For this review, use the dimensioned drawing (mm, ordinates from the lowest corner) and the shaded views. A direction names the side the tool comes from. Round coordinates to 2 decimals unless told otherwise and drop trailing zeros. Order: outer loops, then holes, each group sorted by start corner. A loop starts at its lowest first (then second) coordinate and runs counter-clockwise, first axis right, second up. Notation, with made-up numbers: (2, 18) - (39, 18) arc R29 ccw to (39, 48) - close; hole circle Ø11 at (30.25, -16.75). An arc over 180 degrees is marked (long way). Use CSV: the item, a comma, the result in double quotes. Start each with the question number.
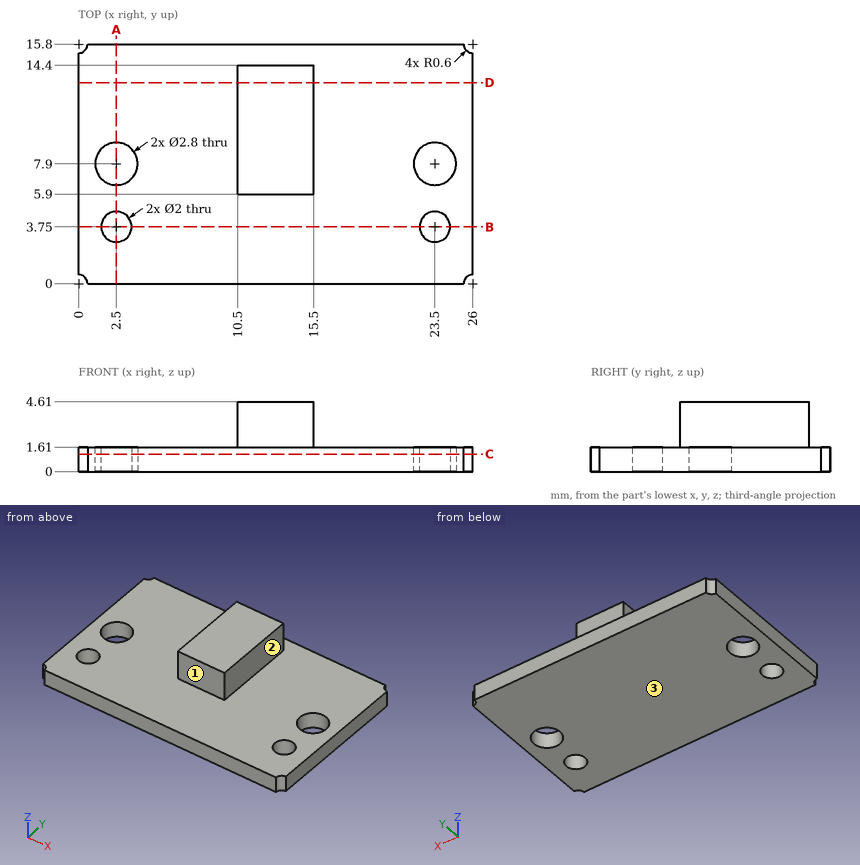
Q1. Take a section at C-C (z = 1.15). State the section outline as (x, y) points, plus the area to 3 significant figures.
Q2. For L1, parallel to Y at x = 23.5, z = 1.35; L2, parallel to Z at x = 5.25, y = 8.5; L3, parallel to X at y = 14, z = 4.3, list the stretches that pass through material, from the lowest coordinate up. Write a range as [from, to].
Q3. Tool access review of the marked faces 1, 2 and 3: name each direction out of +Z, -Z, +X, -X, +Y, -Y from which nothing blocks a thin tool from reaching the whole face with its end or side.
Q4. Clearance check with flat-ended pins moving along their axes: pin 1 (3.5 mm diameter, centred on x = 23.5, y = 7.9, fed in from +Z); pin 2 (2 mm diameter, centred on y = 13.5, z = 2, fed in from -X); pin 3 (2.5 mm diameter, centred on y = 11, z = 3, fed in from +X); pin 4 (0.9 mm diameter, centred on y = 9, z = 4, fed in from -X). State where each tip first meets the part, or that it passes through.
Q5. Take a section at B-B (y = 3.75). State the section outline as (x, z) points, plus the area to 3 significant figures.
Q6. Take a section at D-D (y = 13.25). State the section outline as (x, z) points, plus the area to 3 significant figures.
Q7. Take a section at A-A (x = 2.5). State the section outline as (y, z) points.
Findings below:
1,outline,"(0, 0.6) arc R0.6 cw to (0.6, 0) - (25.4, 0) arc R0.6 cw to (26, 0.6) - (26, 15.2) arc R0.6 cw to (25.4, 15.8) - (0.6, 15.8) arc R0.6 cw to (0, 15.2) - close; hole circle Ø2.8 at (2.5, 7.9); hole circle Ø2 at (2.5, 3.75); hole circle Ø2.8 at (23.5, 7.9); hole circle Ø2 at (23.5, 3.75)"
1,area,"391 mm^2"
2,L1,"y = [0, 2.75], [4.75, 6.5], [9.3, 15.8]"
2,L2,"z = [0, 1.61]"
2,L3,"x = [10.5, 15.5]"
3,face 1,"+Z, +X, -X, -Y"
3,face 2,"+Z, +X, +Y, -Y"
3,face 3,"-Z, +X, -X, +Y, -Y"
4,pin 1,"stops at z = 1.61"
4,pin 2,"stops at x = 0"
4,pin 3,"stops at x = 15.5"
4,pin 4,"stops at x = 10.5"
5,outline,"(0, 0) - (1.5, 0) - (1.5, 1.61) - (0, 1.61) - close; (3.5, 0) - (22.5, 0) - (22.5, 1.61) - (3.5, 1.61) - close; (24.5, 0) - (26, 0) - (26, 1.61) - (24.5, 1.61) - close"
5,area,"35.4 mm^2"
6,outline,"(0, 0) - (26, 0) - (26, 1.61) - (15.5, 1.61) - (15.5, 4.61) - (10.5, 4.61) - (10.5, 1.61) - (0, 1.61) - close"
6,area,"56.9 mm^2"
7,outline,"(0, 0) - (2.75, 0) - (2.75, 1.61) - (0, 1.61) - close; (4.75, 0) - (6.5, 0) - (6.5, 1.61) - (4.75, 1.61) - close; (9.3, 0) - (15.8, 0) - (15.8, 1.61) - (9.3, 1.61) - close"
